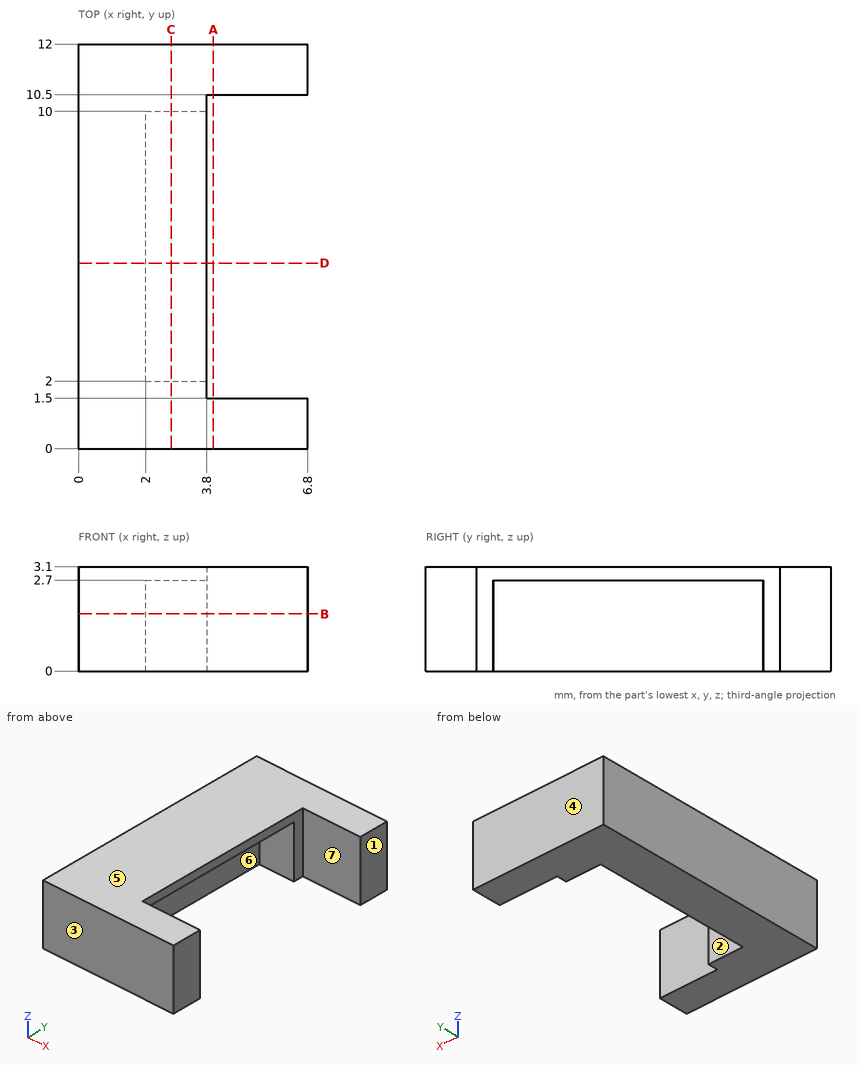
Job drawing, mm, ordinate dimensions from the low corner. One solid piece. A direction names the side the tool comes from. Coordinates: 2 decimals unless noted, no trailing zeros. Order: outer loops, then holes, each group sorted by start corner. A loop starts at its lowest first (then second) coordinate and runs counter-clockwise, first axis right, second up. Notation, with made-up numbers: (-29, 80) -> (-4, 80) arc R16 cw to (-4, 94) -> close; hole circle Ø6 at (81.5, -35.75). An arc over 180 degrees is marked (long way). Answer in a Markdown table with one row per item. Add a question column.
Q1. Band-saw the part on B-B, the plane z = 1.7. List the corners of the cut face in (x, y).
Q2. Drop a flat-ended pin along its axis: pin 1 (1.6 mm diameter, centred on y = 8, z = 1.5, fed in from +X). Give the stop position or say it passes through.
Q3. Mould opens along Y. For the marked faces 1, 2, 3 and 4 say: +Y half, -Y half, draft (parallel to the pull), parting line (faces both ways), or undercut.
Q4. Which spindle directions (+Z, -Z, +X, -X, +Y, -Y) get a long thin tool onto all of the face, cutting with end or side? Do the marked faces 5, 6 and 7. Say none if no direction does.
Q5. Band-saw the part on D-D, the plane y = 5.5. List the corners of the cut face in (x, z), then the cut area to 3 significant figures.
Q6. Band-saw the part on C-C, the plane x = 2.75. List the corners of the cut face in (y, z).
Q7. Band-saw the part on A-A, the plane x = 4. List the corners of the cut face in (y, z), then the cut area to 3 significant figures.
Q8. Wall check: line 1 along Y through (x, z) = (2.75, 2); line 2 along Y through (x, z) = (6.5, 1.1); line 3 along X through (y, z) = (3.5, 0.95). Give the ranges that are in metal, low to high. Write a range as [from, to].
Answers follow:
| question | item | result |
|---|---|---|
| 1 | outline | (0, 0) -> (6.8, 0) -> (6.8, 1.5) -> (3.8, 1.5) -> (3.8, 2) -> (2, 2) -> (2, 10) -> (3.8, 10) -> (3.8, 10.5) -> (6.8, 10.5) -> (6.8, 12) -> (0, 12) -> close |
| 2 | pin 1 | x = 2 |
| 3 | face 1 | draft |
| 3 | face 2 | undercut |
| 3 | face 3 | -Y half |
| 3 | face 4 | +Y half |
| 4 | face 5 | +Z, +X, -X, +Y, -Y |
| 4 | face 6 | -Z, +X |
| 4 | face 7 | +Z, -Z, +X |
| 5 | outline | (0, 0) -> (2, 0) -> (2, 2.7) -> (3.8, 2.7) -> (3.8, 3.1) -> (0, 3.1) -> close |
| 5 | area | 6.92 mm^2 |
| 6 | outline | (0, 0) -> (2, 0) -> (2, 2.7) -> (10, 2.7) -> (10, 0) -> (12, 0) -> (12, 3.1) -> (0, 3.1) -> close |
| 7 | outline | (0, 0) -> (1.5, 0) -> (1.5, 3.1) -> (0, 3.1) -> close; (10.5, 0) -> (12, 0) -> (12, 3.1) -> (10.5, 3.1) -> close |
| 7 | area | 9.30 mm^2 |
| 8 | line 1 | [0, 2], [10, 12] |
| 8 | line 2 | [0, 1.5], [10.5, 12] |
| 8 | line 3 | [0, 2] |
